Geometry check sheet. Reference: drawing and pictorial views, mm from the part's lowest x, y, z. Give positions to 0.01 mm unless a question says otherwise; leave off trailing zeros. Order: outer loops, then holes, each group sorted by start corner. A loop starts at its lowest first (then second) coordinate and runs counter-clockwise, first axis right, second up.
Item 1: Sectioned sample at D-D on z = 2.25. Record the boundary of the cut face in (x, y).
Item 2: Release check for a two-part mould opening along X. For the marked faces 1, 2, 3 and 4 record: released by +X, released by -X, zero draft, split by the parting line, or undercut.
Item 3: Gauge pin test, flat ends, axial feed: P1, Ø4, axis at x = 6, z = 6, coming from the +Y side; P2, Ø1, axis at y = 2, z = 9.5, coming from the -X side; P3, Ø1.5, axis at x = 10, y = 4, coming from the -Z side. Record the tip position at first contact, or that the pin passes through.
Item 4: Material ranges on line 1 along X through (y, z) = (2.85, 6); line 2 along Z through (x, y) = (6.5, 4.85); line 3 along Z through (x, y) = (4.75, 4.85), recorded low to high.
Item 5: Sectioned sample at A-A on z = 6. Record the boundary of the cut face in (x, y), and give its area (3 significant figures).
Item 6: Sectioned sample at C-C on y = 4.05. Record the boundary of the cut face in (x, z).
Item 7: Sectioned sample at B-B on x = 6. Record the boundary of the cut face in (y, z), and give its area (3 significant figures).
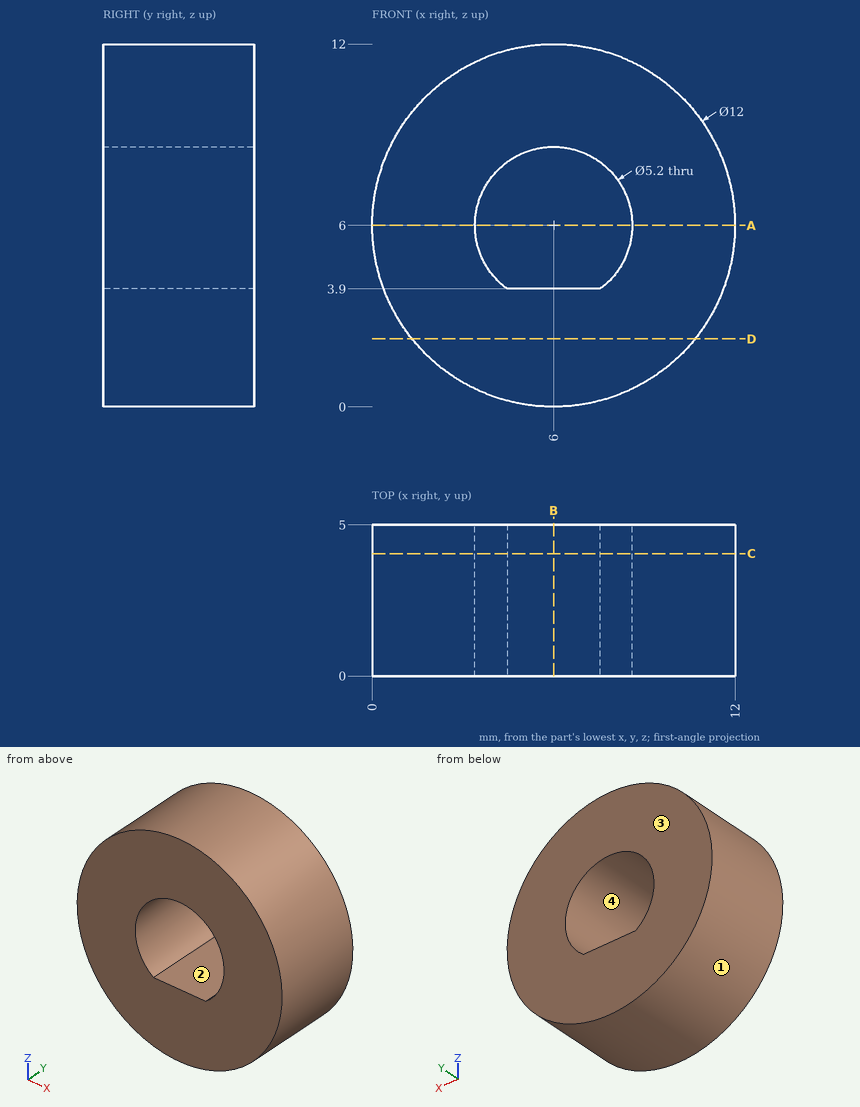
Report:
1. outline: (1.32, 0) - (10.68, 0) - (10.68, 5) - (1.32, 5) - close
2. face 1: split by the parting line
2. face 2: undercut
2. face 3: zero draft
2. face 4: undercut
3. P1: passes through
3. P2: stops at x = 0.8
3. P3: stops at z = 0.96
4. line 1: x = 0 to 3.4, 8.6 to 12
4. line 2: z = 0.02 to 3.9, 8.55 to 11.98
4. line 3: z = 0.13 to 3.9, 8.28 to 11.87
5. outline: (0, 0) - (3.4, 0) - (3.4, 5) - (0, 5) - close; (8.6, 0) - (12, 0) - (12, 5) - (8.6, 5) - close
5. area: 34.0 mm2
6. outline: circle Ø12 at (6, 6); hole (4.47, 3.9) - (7.53, 3.9) arc R2.6 ccw (long way) to start
7. outline: (0, 0) - (5, 0) - (5, 3.9) - (0, 3.9) - close; (0, 8.6) - (5, 8.6) - (5, 12) - (0, 12) - close
7. area: 36.5 mm2
